from build123d import *

# Parameters (mm, degrees)
SKETCH_1_W               = 90
SKETCH_1_H               = 14
EXTRUDE_1_DEPTH          = 4
CHAMFER_1_SIZE           = 2
SKETCH_2_W               = 14
SKETCH_2_H               = 14
EXTRUDE_2_DEPTH          = 17
CUT_EXTRUDE_START        = 2
SKETCH_3_OUTSIDE_W       = 110.694
SKETCH_3_OUTSIDE_H       = 34.694
SKETCH_3_OUTSIDE_W_2     = 12
SKETCH_3_OUTSIDE_H_2     = 12
CUT_EXTRUDE_1_DEPTH      = 6
CHAMFER_2_SIZE           = 2
SKETCH_4_W               = 2
SKETCH_4_H               = 10
EXTRUDE_3_DEPTH          = 2
CUT_EXTRUDE_2_DEPTH      = 51.149775672
CUT_EXTRUDE_2_DEPTH_BACK = 51.149775672
SKETCH_5_R               = 2
CUT_EXTRUDE_3_DEPTH      = 52.019604075
CUT_EXTRUDE_3_DEPTH_BACK = 12
SKETCH_6_R               = 4
CHAMFER_3_SIZE           = 2
SKETCH_7_R               = 3.5
CUT_EXTRUDE_4_DEPTH      = 50.345719166
CUT_EXTRUDE_5_DEPTH      = 52.019604075
CUT_EXTRUDE_5_DEPTH_BACK = 4
SKETCH_8_W               = 2
SKETCH_8_H               = 10


with BuildPart() as part:
    # 草图1 → 凸台-拉伸1 (new body)
    with BuildSketch(Plane(origin=(0, 0, 0), x_dir=(1, 0, 0), z_dir=(0, 1, 0))):
        Rectangle(SKETCH_1_W, SKETCH_1_H)
    extrude(amount=EXTRUDE_1_DEPTH)

    # 倒角1
    chamfer_1_edges = [part.edges().sort_by_distance(p)[0] for p in [
        (45, 2, 7),
        (-45, 2, 7),
        (-45, 2, -7),
        (45, 2, -7),
    ]]
    chamfer(chamfer_1_edges, length=CHAMFER_1_SIZE)

    # 草图2 → 凸台-拉伸2 (add)
    with BuildSketch(Plane(origin=(0, 4, 0), x_dir=(1, 0, 0), z_dir=(0, 1, 0))):
        Rectangle(SKETCH_2_W, SKETCH_2_H)
    extrude(amount=EXTRUDE_2_DEPTH)

    # 草图3 outside → 切除-拉伸1 (cut)
    with BuildSketch(Plane(origin=(0, 4, 0), x_dir=(1, 0, 0), z_dir=(0, 1, 0)).offset(CUT_EXTRUDE_START)):
        Rectangle(SKETCH_3_OUTSIDE_W, SKETCH_3_OUTSIDE_H)
        Rectangle(SKETCH_3_OUTSIDE_W_2, SKETCH_3_OUTSIDE_H_2, mode=Mode.SUBTRACT)
    extrude(amount=CUT_EXTRUDE_1_DEPTH, mode=Mode.SUBTRACT)

    # 倒角2
    chamfer_2_edges = [part.edges().sort_by_distance(p)[0] for p in [
        (7, 16.5, 7),
        (7, 16.5, -7),
        (-7, 16.5, -7),
        (-7, 16.5, 7),
        (-7, 5, 7),
        (-7, 5, -7),
        (7, 5, -7),
        (7, 5, 7),
        (6, 9, -6),
        (-6, 9, -6),
        (-6, 9, 6),
        (6, 9, 6),
    ]]
    chamfer(chamfer_2_edges, length=CHAMFER_2_SIZE)

    # 草图4 → 凸台-拉伸3 (add)
    with BuildSketch(Plane(origin=(0, 21, 0), x_dir=(1, 0, 0), z_dir=(0, 1, 0))):
        with Locations((-6, 0)):
            Rectangle(SKETCH_4_W, SKETCH_4_H)
    extrude_3 = extrude(amount=EXTRUDE_3_DEPTH)

    # 镜向1: 凸台-拉伸3 across plane
    add(extrude_3.mirror(Plane(origin=(0, 0, 0), x_dir=(0, 0, 1), z_dir=(1, 0, 0))))

    # 草图5 → 切除-拉伸2 (cut, two sides: drawn at the far end of the back side and taken through both)
    with BuildSketch(Plane(origin=(0, 21, 0), x_dir=(1, 0, 0), z_dir=(0, 1, 0)).offset(-CUT_EXTRUDE_2_DEPTH_BACK)):
        with Locations(Location((0, 0, 0), (0, 0, 270))):
            Circle(SKETCH_5_R)
    extrude(amount=CUT_EXTRUDE_2_DEPTH + CUT_EXTRUDE_2_DEPTH_BACK, mode=Mode.SUBTRACT)

    # 草图6 → 切除-拉伸3 (cut, two sides: drawn at the far end of the back side and taken through both)
    with BuildSketch(Plane.XZ.offset(-CUT_EXTRUDE_3_DEPTH_BACK)):
        with Locations(Location((0, 0, 0), (0, 0, 270))):
            Circle(SKETCH_6_R)
    extrude(amount=CUT_EXTRUDE_3_DEPTH + CUT_EXTRUDE_3_DEPTH_BACK, mode=Mode.SUBTRACT)

    # 倒角3
    chamfer_3_edges = [part.edges().sort_by_distance(p)[0] for p in [
        (0, 12, -2),
    ]]
    chamfer(chamfer_3_edges, length=CHAMFER_3_SIZE - 0.0001)  # a hair under: the kernel refuses the full size

    # 草图7 → 切除-拉伸4 (cut, symmetric)
    with BuildSketch(Plane(origin=(0, 4, 0), x_dir=(1, 0, 0), z_dir=(0, 1, 0))):
        with Locations(Location((-38, 0, 0), (0, 0, 270))):
            Circle(SKETCH_7_R)
    cut_extrude_4 = extrude(amount=CUT_EXTRUDE_4_DEPTH, both=True, mode=Mode.SUBTRACT)

    # 镜向2: 切除-拉伸4 across plane
    add(cut_extrude_4.mirror(Plane(origin=(0, 0, 0), x_dir=(0, 0, 1), z_dir=(1, 0, 0))), mode=Mode.SUBTRACT)

    # 草图8 → 切除-拉伸5 (cut, two sides: drawn at the far end of the back side and taken through both)
    with BuildSketch(Plane(origin=(0, 23, 0), x_dir=(1, 0, 0), z_dir=(0, 1, 0)).offset(-CUT_EXTRUDE_5_DEPTH_BACK)):
        with Locations((6, 0)):
            Rectangle(SKETCH_8_W, SKETCH_8_H)
        with Locations((-6, 0)):
            Rectangle(SKETCH_8_W, SKETCH_8_H)
    extrude(amount=CUT_EXTRUDE_5_DEPTH + CUT_EXTRUDE_5_DEPTH_BACK, mode=Mode.SUBTRACT)


solid = part.part
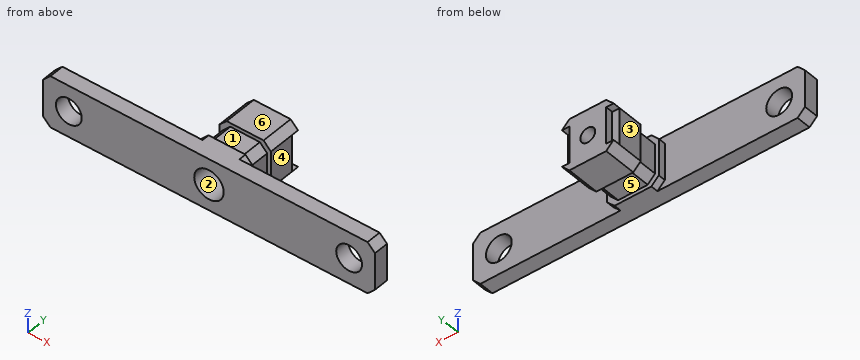
Design review of the part built by this model. Coordinates are the model's own, in mm. Face numbers are marked on the shaded views. A direction names the side the tool comes from. Round coordinates to 2 decimals unless told otherwise and drop trailing zeros. Loops run counter-clockwise (first coordinate to the right, second up) from the corner with the lowest first, then second, coordinate; pieces in that order, holes last. Notation, with made-up numbers: M 43.25,-8.75 L 53.25,-8.75 A7 ccw 53.25,-1.75 Z; hole C 7,-16 d5. An arc over 180 degrees is marked long. Answer as a JSON object with one key per item and string values.
Item 1: The part is to be moulded in two halves that separate along Z. For the marked faces 1, 2 and 3, say which applies: pulls with the +Z half, pulls with the -Z half, needs draft (parallel to the pull), parting line crosses it, or undercut.
Answer sheet:
{"face 1": "pulls with the +Z half", "face 2": "undercut", "face 3": "needs draft"}
Item 2: Clearance check with flat-ended pins moving along their axes: P1, Ø1.6, axis at y = 5.5, z = -0.5, coming from the -X side; P2, Ø0.6, axis at y = 4.5, z = 2, coming from the +X side; P3, Ø1, axis at x = -6, z = 1, coming from the +Y side. State where each tip first meets the part, or that it passes through.
Answer sheet:
{"P1": "stops at x = -7", "P2": "stops at x = 7", "P3": "stops at y = 19"}
Item 3: Wall thickness on L1, parallel to X at y = 2.7, z = 0; L2, parallel to X at y = 19.75, z = 0; L3, parallel to Z at x = 0, y = 8.5: over which ranges is each line inside the solid? List them lowest first. Write a range as from..to.
Answer sheet:
{"L1": "x = -45..-41.5, -34.5..-4, 4..34.5, 41.5..45", "L2": "x = -5..-2, 2..5", "L3": "z = -6..-4, 4..6"}
Item 4: We need section C-C on y = 17.25. Give the boundary of the cut face in (x, z), and give its area (3 significant figures).
Answer sheet:
{"outline": "M -7,-5 L -5,-7 L 5,-7 L 7,-5 L 7,5 L 5,7 L -5,7 L -7,5 Z; hole C 0,0 d4", "area": "175 mm^2"}
Item 5: We need section D-D on x = -38. Give the boundary of the cut face in (y, z).
Answer sheet:
{"outline": "M 0,-7 L 4,-7 L 4,-3.5 L 0,-3.5 Z; M 0,3.5 L 4,3.5 L 4,7 L 0,7 Z"}
Item 6: Machinability: for the marked faces 4, 5 and 6, which of the approach directions +Z, -Z, +X, -X, +Y, -Y give a long, thin tool a straight path to every point of the face, cutting with its end or side? Answer none if there is none.
Answer sheet:
{"face 4": "+Z, -Z, +X, +Y", "face 5": "-Z, +X, -X", "face 6": "+Z, +X, -X, +Y, -Y"}
Item 7: We need section B-B on y = 2.5. Give the boundary of the cut face in (x, z).
Answer sheet:
{"outline": "M -45,-5 L -43,-7 L 43,-7 L 45,-5 L 45,5 L 43,7 L -43,7 L -45,5 Z; hole C -38,0 d7; hole C 0,0 d8; hole C 38,0 d7"}
